Model file for the job. Use its own axes, mm. Face numbers are marked on the shaded views. A direction names the side the tool comes from. Give positions to 0.01 mm unless a question says otherwise; leave off trailing zeros. Write each loop counter-clockwise with the first axis right and the second up, starting at its lowest first coordinate (ties: lowest second). Pieces come first, ordered by that corner, then holes. Notation, with made-up numbers: (-20.75, 17) - (-8.75, 17) arc R23 ccw to (-8.75, 30) - close; hole circle Ø8 at (63.25, 76.5). An arc over 180 degrees is marked (long way). One line per item, written item: value. Start each with the question number.
(1) 3-axis set-ups, long thin cutter, end or side, ignore diameter. For the marked faces 1, 2, 3 and 4: which of +Z, -Z, +X, -X, +Y, -Y reach the whole face in a straight line?
(2) Drop flat-ended pins along their axis: P1, Ø6.5, axis at y = 36, z = 1, coming from the -X side; P2, Ø1.8, axis at y = 33.5, z = 0, coming from the +X side; P3, Ø3, axis at x = 0, y = 21, coming from the +Z side; P4, Ø3.5, axis at x = 0, z = 0, coming from the +Y side. Give the stop position or say it passes through.
(3) Mould opens along Z. For the marked faces 5, 6, 7 and 8 say: pulls with the +Z half, pulls with the -Z half, needs draft (parallel to the pull), parting line crosses it, or undercut.
(4) Cut at C-C, the plane y = 54.5. List the corners of the cut face in (x, z), and give its area (3 significant figures).
(5) Cut at B-B, the plane z = 0. List the corners of the cut face in (x, y).
(6) Cut at A-A, the plane x = 0. List the corners of the cut face in (y, z).
(7) Probe L1, parallel to X at y = 42.5, z = 0; L2, parallel to Z at x = 6, y = 19.5. List the from-to ranges inside material, lowest first.
from build123d import *

# Parameters (mm, degrees)
SKETCH1_W    = 20
SKETCH1_H    = 20
BODY_DEPTH   = 68
SKETCH2_R    = 2.75
SKETCH2_W    = 6
SKETCH2_H    = 5.5
SKETCH2_W_2  = 5.5
SKETCH2_H_2  = 6
PROFIL_DEPTH = 70.455021417


with BuildPart() as part:
    # Sketch1 → Body (new body)
    with BuildSketch(Plane(origin=(0, 0, 0), x_dir=(1, 0, 0), z_dir=(0, 1, 0))):
        Rectangle(SKETCH1_W, SKETCH1_H)
    extrude(amount=BODY_DEPTH)

    # Sketch2 → Profil (cut, through all)
    with BuildSketch(Plane(origin=(0, 68, 0), x_dir=(1, 0, 0), z_dir=(0, 1, 0))):
        with Locations(Location((0, 0, 0), (0, 0, 270))):
            Circle(SKETCH2_R)
        with Locations((0, 7.25)):
            Rectangle(SKETCH2_W, SKETCH2_H)
        with Locations((7.25, 0)):
            Rectangle(SKETCH2_W_2, SKETCH2_H_2)
        with Locations((0, -7.25)):
            Rectangle(SKETCH2_W, SKETCH2_H)
        with Locations((-7.25, 0)):
            Rectangle(SKETCH2_W_2, SKETCH2_H_2)
    extrude(amount=-PROFIL_DEPTH, mode=Mode.SUBTRACT)


solid = part.part
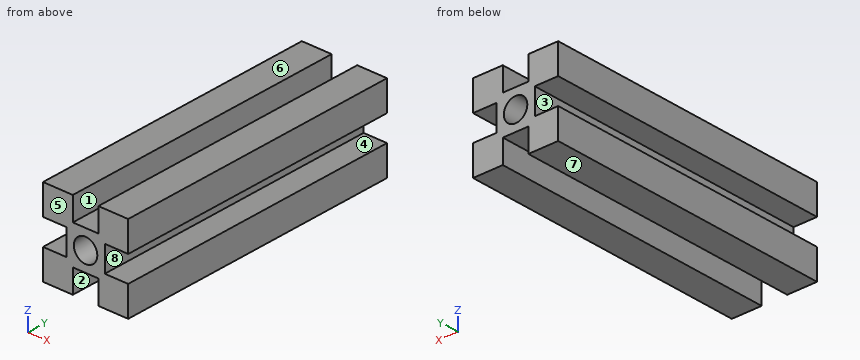
Answers follow:
1. face 1: +Z, +Y, -Y
1. face 2: -Z, +Y, -Y
1. face 3: -X, +Y, -Y
1. face 4: +X, +Y, -Y
2. P1: stops at x = -10
2. P2: stops at x = 4.5
2. P3: stops at z = 4.5
2. P4: passes through
3. face 5: needs draft
3. face 6: pulls with the +Z half
3. face 7: pulls with the -Z half
3. face 8: undercut
4. outline: (-10, -10) - (-3, -10) - (-3, -4.5) - (3, -4.5) - (3, -10) - (10, -10) - (10, -3) - (4.5, -3) - (4.5, 3) - (10, 3) - (10, 10) - (3, 10) - (3, 4.5) - (-3, 4.5) - (-3, 10) - (-10, 10) - (-10, 3) - (-4.5, 3) - (-4.5, -3) - (-10, -3) - close; hole circle Ø5.5 at (0, 0)
4. area: 244 mm²
5. outline: (-4.5, 0) - (-2.75, 0) - (-2.75, 68) - (-4.5, 68) - close; (2.75, 0) - (4.5, 0) - (4.5, 68) - (2.75, 68) - close
6. outline: (0, -4.5) - (68, -4.5) - (68, -2.75) - (0, -2.75) - close; (0, 2.75) - (68, 2.75) - (68, 4.5) - (0, 4.5) - close
7. L1: x = -4.5 to -2.75, 2.75 to 4.5
7. L2: z = -10 to -3, 3 to 10
